Verification items for this drawing (mm, ordinates from the low corner). Round coordinates to 2 decimals unless told otherwise and drop trailing zeros. Loops run counter-clockwise (first coordinate to the right, second up) from the corner with the lowest first, then second, coordinate; pieces in that order, holes last. Notation, with made-up numbers: (-3.5, 61.5) -> (36.5, 61.5) arc R15 ccw to (36.5, 79.5) -> close; hole circle Ø7 at (-31.5, 19). An arc over 180 degrees is marked (long way). Use a Markdown table: item, result. Add a question column.
Q1. Material ranges on L1, parallel to Z at x = 2, y = 1.55, recorded low to high.
Q2. Gauge pin test, flat ends, axial feed: P1, Ø2, axis at x = 29.5, y = 2.5, coming from the +Z side; P2, Ø2, axis at y = 1.5, z = 129, coming from the -X side; P3, Ø2, axis at x = 39.5, y = 2, coming from the -Z side. Record the tip position at first contact, or that the pin passes through.
Q3. Sectioned sample at B-B, the plane x = 4.5. Enter the section's corners in (y, z).
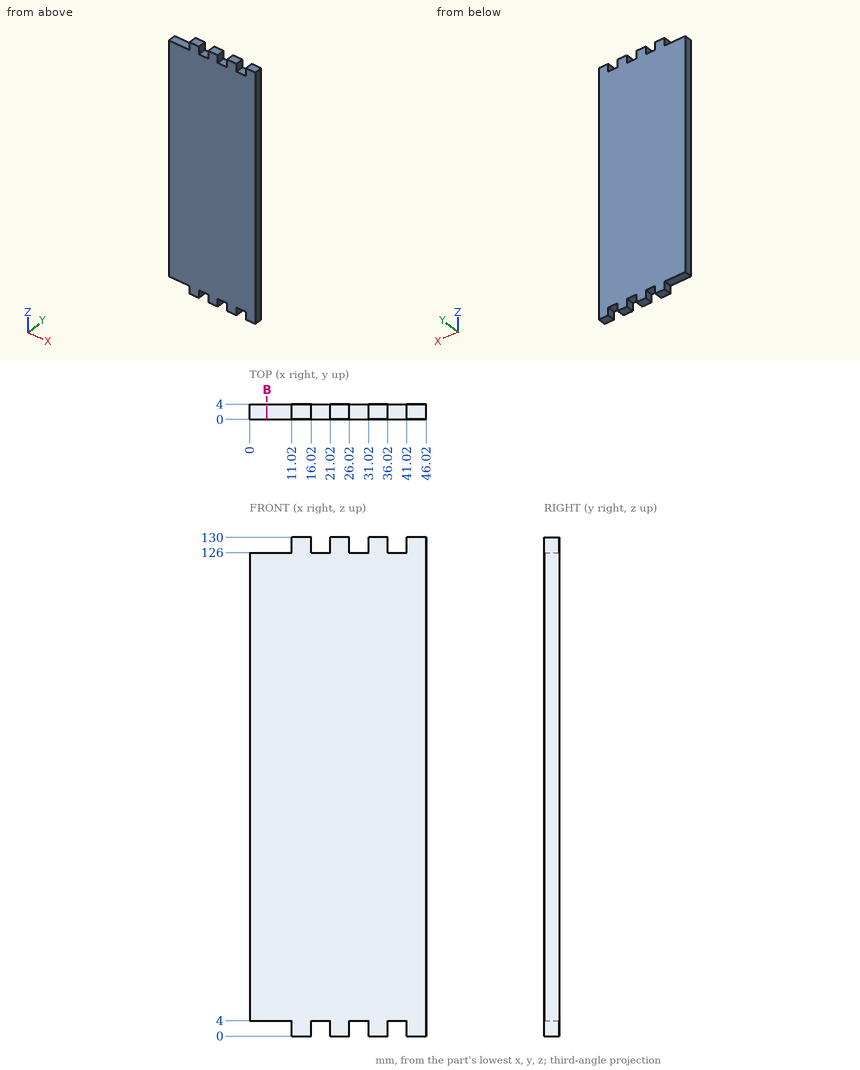
Values:
| question | item | result |
|---|---|---|
| 1 | L1 | 4 to 126 |
| 2 | P1 | z = 126 |
| 2 | P2 | x = 11.02 |
| 2 | P3 | z = 4 |
| 3 | outline | (0, 4) -> (4, 4) -> (4, 126) -> (0, 126) -> close |
